Can you work these out from the drawing? Everything is in mm from the part's minimum corner. A direction names the side the tool comes from. Coordinates: 2 decimals unless noted, no trailing zeros. Loops run counter-clockwise (first coordinate to the right, second up) from the corner with the lowest first, then second, coordinate; pieces in that order, holes last. Notation, with made-up numbers: (-39.5, 69.25) - (-31.5, 69.25) arc R15 ccw to (-31.5, 86.25) - close; hole circle Ø8 at (-13, -6). An arc over 180 degrees is marked (long way). One line per question, with ' | ' between items. Start each with the question number.
1. I want a section at A-A, the plane y = 5.2. Write out the boundary of the cut face in (x, z), then the cut area to 3 significant figures.
2. I want a section at B-B, the plane z = 2.5. Write out the boundary of the cut face in (x, y), then the cut area to 3 significant figures.
3. Which directions (+Z, -Z, +X, -X, +Y, -Y) give clear straight access to the entire face, cutting with the end or side of a thin tool? Please do the marked faces 4 and 5.
4. We'd pull the mould along Y, two halves only. Please class the marked faces 1, 2 and 3: pulls with the +Y half, pulls with the -Y half, needs draft (parallel to the pull), parting line crosses it, or undercut.
5. I want a section at D-D, the plane y = 24.25. Write out the boundary of the cut face in (x, z).
6. I'm going to push flat-ended pins straight in: P1, Ø8, axis at y = 2.5, z = 5.5, coming from the +X side; P2, Ø3, axis at x = 12, z = 4, coming from the -Y side; P3, Ø3, axis at x = 9, y = 5.2, coming from the +Z side. Where does each tip first touch, or does it pass through?
7. Please list where these lines run through material, in increasing order: L1, parallel to X at y = 18.25, z = 5.5; L2, parallel to Z at x = 1.5, y = 6; L3, parallel to Y at x = 9, z = 10.75. Write a range as [from, to].
8. I want a section at C-C, the plane x = 9. Write out the boundary of the cut face in (y, z).
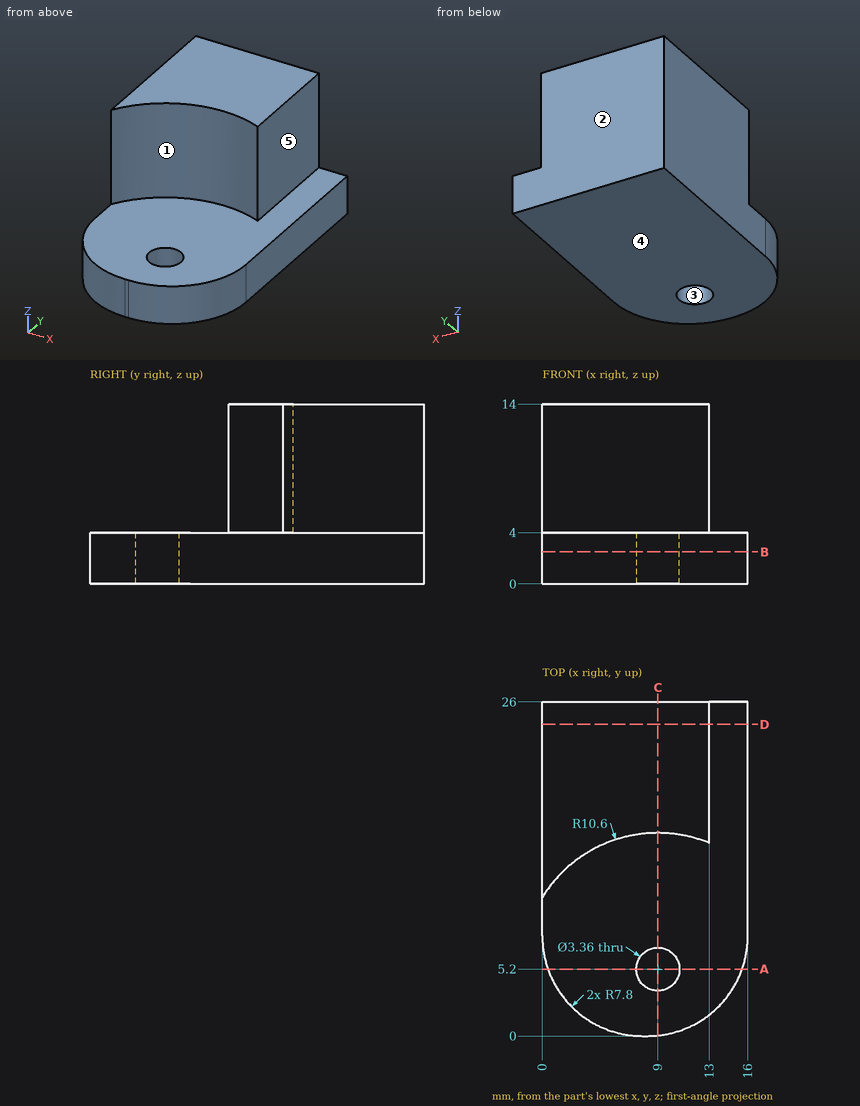
Results are:
1) outline: (0.45, 0) - (7.32, 0) - (7.32, 4) - (0.45, 4) - close; (10.68, 0) - (15.55, 0) - (15.55, 4) - (10.68, 4) - close | area: 47.0 mm2
2) outline: (0, 7.8) arc R7.8 ccw to (7.8, 0) - (8.2, 0) arc R7.8 ccw to (16, 7.8) - (16, 26) - (0, 26) - close; hole circle Ø3.36 at (9, 5.2) | area: 381 mm2
3) face 4: -Z, +X, -X, +Y, -Y | face 5: +Z, +X, +Y, -Y
4) face 1: pulls with the -Y half | face 2: pulls with the +Y half | face 3: undercut
5) outline: (0, 0) - (16, 0) - (16, 4) - (13, 4) - (13, 14) - (0, 14) - close
6) P1: stops at x = 15.84 | P2: stops at y = 0.35 | P3: passes through
7) L1: x = [0, 13] | L2: z = [0, 4] | L3: y = [15.8, 26]
8) outline: (0.04, 0) - (3.52, 0) - (3.52, 4) - (0.04, 4) - close; (6.88, 0) - (26, 0) - (26, 14) - (15.8, 14) - (15.8, 4) - (6.88, 4) - close
